Part model, mm, in its own coordinate system. A direction names the side the tool comes from. Give positions to 0.01 mm unless a question says otherwise; leave off trailing zeros. Order: outer loops, then holes, each group sorted by start corner. A loop starts at its lowest first (then second) coordinate and runs counter-clockwise, first axis right, second up. Notation, with made-up numbers: (9, 57.25) - (42, 57.25) arc R30 cw to (42, 96.25) - close; hole circle Ø6 at (-3, 8). An arc over 180 degrees is marked (long way). One line per item, written item: value.
```python
from build123d import *

# Parameters (mm, degrees)
SKETCH1_R                               = 20
BOSS_EXTRUDE1_DEPTH                     = 20
CBORE_FOR_M5_HEX_HEAD_BOLT5_D           = 5.5
CBORE_FOR_M5_HEX_HEAD_BOLT5_CBORE_D     = 10
CBORE_FOR_M5_HEX_HEAD_BOLT5_CBORE_DEPTH = 5


with BuildPart() as part:
    # Sketch1 → Boss-Extrude1 (new body)
    with BuildSketch(Plane(origin=(0, 0, 0), x_dir=(1, 0, 0), z_dir=(0, 1, 0))):
        Circle(SKETCH1_R)
    extrude(amount=BOSS_EXTRUDE1_DEPTH)

    # CBORE for M5 Hex Head Bolt5 (through all)
    with Locations(Plane(origin=(0, 20, -12), x_dir=(0, 0, 1), z_dir=(0, 1, 0))):
        with Locations((0, 0), (12, 12), (24, 0), (12, -12)):
            CounterBoreHole(CBORE_FOR_M5_HEX_HEAD_BOLT5_D / 2, CBORE_FOR_M5_HEX_HEAD_BOLT5_CBORE_D / 2, CBORE_FOR_M5_HEX_HEAD_BOLT5_CBORE_DEPTH)


solid = part.part
```
1) Pin check, flat tips, straight feed: pin 1 (12 mm diameter, centred on y = 6, z = 15, fed in from -X); pin 2 (1 mm diameter, centred on y = 5.5, z = -10, fed in from +X); pin 3 (5 mm diameter, centred on x = -12, z = 0, fed in from +Y) (3 decimals); pin 4 (10 mm diameter, centred on x = 8, y = 6.5, fed in from +Z). Stop position of each tip, or through.
Outcome:
pin 1: stops at x = -17.86
pin 2: stops at x = 17.6
pin 3: passes through
pin 4: stops at z = 19.77
2) Cut at D-D, the plane x = 0. Give the cut face in (y, z).
Outcome:
outline: (0, -20) - (20, -20) - (20, -17) - (15, -17) - (15, -14.75) - (0, -14.75) - close; (0, -9.25) - (15, -9.25) - (15, -7) - (20, -7) - (20, 7) - (15, 7) - (15, 9.25) - (0, 9.25) - close; (0, 14.75) - (15, 14.75) - (15, 17) - (20, 17) - (20, 20) - (0, 20) - close
3) Which spindle directions (+Z, -Z, +X, -X, +Y, -Y) get a long thin tool onto all of the face, cutting with end or side? Do faces 4 (the flat face through (-2.2, 15, -9.8)), 5 (the cylindrical face through (13.859, 7.395, 2.027)). Say none if no direction does.
Outcome:
face 4: +Y
face 5: +Y, -Y
4) Cut at B-B, the plane x = 12. Give the cut face in (y, z).
Outcome:
outline: (0, -16) - (20, -16) - (20, -5) - (15, -5) - (15, -2.75) - (0, -2.75) - close; (0, 2.75) - (15, 2.75) - (15, 5) - (20, 5) - (20, 16) - (0, 16) - close
5) Cut at A-A, the plane z = 12. Give the cut face in (x, y), then the cut area to 4 significant figures.
Outcome:
outline: (-16, 0) - (-2.75, 0) - (-2.75, 15) - (-5, 15) - (-5, 20) - (-16, 20) - close; (2.75, 0) - (16, 0) - (16, 20) - (5, 20) - (5, 15) - (2.75, 15) - close
area: 507.5 mm^2
6) Cut at C-C, the plane z = 0. Give the cut face in (x, y), then the cut area to 3 significant figures.
Outcome:
outline: (-20, 0) - (-14.75, 0) - (-14.75, 15) - (-17, 15) - (-17, 20) - (-20, 20) - close; (-9.25, 0) - (9.25, 0) - (9.25, 15) - (7, 15) - (7, 20) - (-7, 20) - (-7, 15) - (-9.25, 15) - close; (14.75, 0) - (20, 0) - (20, 20) - (17, 20) - (17, 15) - (14.75, 15) - close
area: 535 mm^2
7) Drill centre lines: line 1 along X through (y, z) = (18.7, 0); line 2 along X through (y, z) = (3.25, -1). Where is each one in solid material? Low to high. Write a range as from..to.
Outcome:
line 1: x = -20..-17, -7..7, 17..20
line 2: x = -19.97..-14.56, -9.44..9.44, 14.56..19.97
8) Mould opens along Z. For faces 1 (the flat face through (0, 20, 0)), 2 (the cylindrical face through (-4.336, 9.86, 19.524)), 3 (the cylindrical face through (-7.043, 17.535, -0.651)) say: released by +Z, released by -Z, zero draft, split by the parting line, or undercut.
Outcome:
face 1: zero draft
face 2: split by the parting line
face 3: undercut
